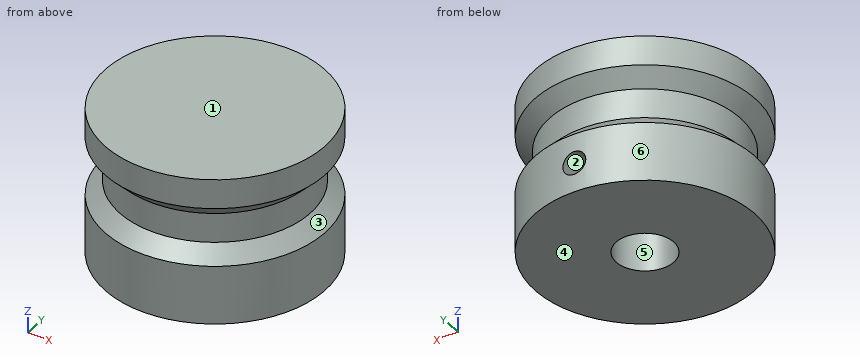
Autodesk Inventor part; units mm, degrees
ref_plane "Work Plane1" through (0, 9.525, -10.16) normal (0, 1, 0) x (-1, 0, 0)
ref_plane "YZ Plane" through (0, 0, 0) normal (1, 0, 0) x (0, 1, 0)
ref_plane "XY Plane" through (0, 0, 0) normal (0, 0, 1) x (1, 0, 0)
sketch "Sketch1" plane through (0, 0, 0) normal (1, 0, 0) x (0, 1, 0)
  line L0 (0, 0) -> (9.525, 0)
  line L1 (9.525, 0) -> (9.525, -2.54)
  line L2 (9.525, -2.54) -> (8.255, -3.81)
  line L3 (8.255, -3.81) -> (8.255, -6.35)
  line L4 (8.255, -6.35) -> (9.525, -7.62)
  line L5 (9.525, -7.62) -> (9.525, -12.7)
  line L6 (9.525, -12.7) -> (0, -12.7)
  line L7 (0, -12.7) -> (0, 0)
  line L8 (0, -15.24) -> (0, 2.54)
  dimension "d0" = 9.525
  dimension "d1" = 135
  dimension "d2" = 2.54
  dimension "d4" = 1.27
  dimension "d5" = 12.7
  dimension "d7" = 2.54
revolve "Revolution1" add sketch "Sketch1" angle 360 about axis through (0, 0, -10) along (0, 0, 1)
sketch "Sketch2" plane through (0, 0, -12.7) normal (0, 0, -1) x (-1, 0, 0)
  circle A0 centre (0, 0) radius 9.525
hole "Hole1" at (0, 0, -12.7) direction (0, 0, 1) diameter 5 depth 11.1125 tip angle 118
ref_plane "Work Plane1" through (0, 9.525, -10.16) normal (0, 1, 0) x (-1, 0, 0)
sketch "Sketch3" plane through (0, 9.525, -10.16) normal (0, 1, 0) x (-1, 0, 0)
  line L0 (0, 10.16) -> (0, 0) construction
  dimension "d16" = 10.16
hole "Hole2" at (0, 9.525, -10.16) direction (0, -1, 0) diameter 2 end up to surface
properties part number "wheel_hub"
Check sheet for the modelled part. Datum: model origin and axes. Units: mm. Face numbers are marked on the shaded views. A direction names the side the tool comes from. Round coordinates to 2 decimals unless told otherwise and drop trailing zeros. Loops run counter-clockwise (first coordinate to the right, second up) from the corner with the lowest first, then second, coordinate; pieces in that order, holes last.
1. Set-up check for the marked faces 1, 2 and 3: record each of +Z, -Z, +X, -X, +Y, -Y from which the full face is reachable in a straight line by a thin tool's end or side.
2. Gauge pin test, flat ends, axial feed: pin 1 Ø6 at (x, y) = (0, 0) entering from +Z; pin 2 Ø1 at (x, z) = (-5, -4.5) entering from -Y; pin 3 Ø6 at (x, z) = (-6, -2.5) entering from -Y; pin 4 Ø2 at (y, z) = (-5.5, -5.5) entering from -X. Record the tip position at first contact, or that the pin passes through.
3. Sectioned sample at C-C on z = -10. Record the boundary of the cut face in (x, y) (3 decimals), and give its area (3 significant figures).
4. Sectioned sample at A-A on z = -8.25. Record the boundary of the cut face in (x, y) (3 decimals).
5. Sectioned sample at B-B on z = -4.25. Record the boundary of the cut face in (x, y) (3 decimals), and give its area (3 significant figures).
6. Mould release check, pull along Y, two halves, no side actions. Record for the marked faces 4, 5 and 6: released by +Y, released by -Y, zero draft, split by the parting line, or undercut.
7. Scan lines: probe 1 along Y at (x, z) = (0, -5.25) (3 decimals); probe 2 along Y at (x, z) = (0, -8.5) (3 decimals). Record each from-to range of solid material in increasing order.
Recorded:
1. face 1: +Z, +X, -X, +Y, -Y
1. face 2: +Y
1. face 3: none
2. pin 1: stops at z = 0
2. pin 2: stops at y = -6.92
2. pin 3: stops at y = -9.04
2. pin 4: stops at x = -6.92
3. outline: (-0.987, 2.297) - (-0.987, 9.474) arc R9.525 ccw (long way) to (0.987, 9.474) - (0.987, 2.297) arc R2.5 cw (long way) to start
3. area: 251 mm2
4. outline: circle Ø19.05 at (0, 0); hole circle Ø5 at (0, 0)
5. outline: circle Ø16.51 at (0, 0); hole circle Ø5 at (0, 0)
5. area: 194 mm2
6. face 4: zero draft
6. face 5: undercut
6. face 6: split by the parting line
7. probe 1: y = -8.255 to -2.5, 2.5 to 8.255
7. probe 2: y = -9.525 to -2.5, 2.5 to 9.525
